Source: CAD feature listing. Evaluate the final solid. Frame: model axes, mm. Face numbers are marked on the shaded views. Give positions to 0.01 mm unless a question says otherwise; leave off trailing zeros. Order: outer loops, then holes, each group sorted by start corner. A loop starts at its lowest first (then second) coordinate and runs counter-clockwise, first axis right, second up.
from build123d import *

# Parameters (mm, degrees)
F0_R     = 1.2342692754
F0_R_2   = 1.7514332525
F0_R_3   = 1.6840139575
F0_R_4   = 0.6424379712
F0_R_5   = 0.6344814838
F1_DEPTH = 3.302


with BuildPart() as f1:
    # F0 (on Right) → F1 (new body)
    with BuildSketch(Plane.YZ):
        Polygon((30.1141384989, 0), (0, 0), (-32.9401008785, 0), (-32.9401008785, -0.8831103914), (-32.9401008785, -2.5610264856), (-32.9401008785, -3.4441391472), (-6.9765895605, -5.3869867697), (30.1141384989, -3.6207614467), (30.1141384989, -2.5610264856), (30.1141384989, -0.883640887), align=None)
        with Locations((-23.4924610704, -2.4733557366)):
            Circle(F0_R, mode=Mode.SUBTRACT)
        with Locations((-2.4024450686, -2.4733557366)):
            Circle(F0_R_2, mode=Mode.SUBTRACT)
        with Locations((3.7611864973, -2.4733557366)):
            Circle(F0_R_3, mode=Mode.SUBTRACT)
        Polygon((-32.9401008785, -2.5610264856), (-32.9401008785, -0.8831103914), (-35.3245027363, -0.8831103914), (-35.3245027363, -1.5608620106), (-35.3245027363, -1.7220684385), (-35.3245027363, -1.8952260725), (-35.3245027363, -2.5610264856), align=None)
        Polygon((32.4102304876, -0.883640887), (30.1141384989, -0.883640887), (30.1141384989, -2.5610264856), (32.4102304876, -2.5610264856), (32.4102304876, -1.8952260725), (32.4102304876, -1.7223336863), (32.4102304876, -1.5608620106), align=None)
        with BuildLine():
            Line((-35.3245027363, -1.7220684385), (-35.3245027363, -1.5608620106))
            Line((-35.3245027363, -1.5608620106), (-36.7480435846, -1.5608620106))
            ThreePointArc((-36.7480435846, -1.5608620106), (-36.7395622808, -1.6412672061), (-36.736718196, -1.7220684385))
            Line((-36.736718196, -1.7220684385), (-35.3245027363, -1.7220684385))
        make_face()
        with BuildLine():
            Line((34.18918825, -1.5608620106), (32.4102304876, -1.5608620106))
            Line((32.4102304876, -1.5608620106), (32.4102304876, -1.7223336863))
            Line((32.4102304876, -1.7223336863), (32.4102304876, -1.8952260725))
            Line((32.4102304876, -1.8952260725), (34.1978147229, -1.8702070236))
            ThreePointArc((34.1978147229, -1.8702070236), (34.1834682887, -1.7158143054), (34.18918825, -1.5608620106))
        make_face()
        with BuildLine():
            Line((-36.7497117243, -1.8952260725), (-35.3245027363, -1.8952260725))
            Line((-35.3245027363, -1.8952260725), (-35.3245027363, -1.7220684385))
            Line((-35.3245027363, -1.7220684385), (-36.736718196, -1.7220684385))
            ThreePointArc((-36.736718196, -1.7220684385), (-36.7367181732, -1.7222010624), (-36.7367181656, -1.7223336863))
            ThreePointArc((-36.7367181656, -1.7223336863), (-36.7399711292, -1.8090236652), (-36.7497117243, -1.8952260725))
        make_face()
        with BuildLine():
            ThreePointArc((-36.736718196, -1.7220684385), (-36.7395622808, -1.6412672061), (-36.7480435846, -1.5608620106))
            ThreePointArc((-36.7480435846, -1.5608620106), (-39.050204678, -1.7165627393), (-36.7497117243, -1.8952260725))
            ThreePointArc((-36.7497117243, -1.8952260725), (-36.7399711292, -1.8090236652), (-36.7367181656, -1.7223336863))
            ThreePointArc((-36.7367181656, -1.7223336863), (-36.7367181732, -1.7222010624), (-36.736718196, -1.7220684385))
        make_face()
        with Locations((-37.8934686196, -1.7223336863)):
            Circle(F0_R_4, mode=Mode.SUBTRACT)
        with BuildLine():
            Line((34.1978147229, -1.5608620106), (34.18918825, -1.5608620106))
            ThreePointArc((34.18918825, -1.5608620106), (34.1834682887, -1.7158143054), (34.1978147229, -1.8702070236))
            Line((34.1978147229, -1.8702070236), (34.1978147229, -1.5608620106))
        make_face()
        with BuildLine():
            ThreePointArc((36.5784095148, -1.6824278282), (35.4415677285, -0.4862718496), (34.18918825, -1.5608620106))
            Line((34.18918825, -1.5608620106), (34.1978147229, -1.5608620106))
            Line((34.1978147229, -1.5608620106), (34.1978147229, -1.8702070236))
            ThreePointArc((34.1978147229, -1.8702070236), (35.4748874223, -2.876422446), (36.5784095148, -1.6824278282))
        make_face()
        with Locations((35.3807061911, -1.6824278282)):
            Circle(F0_R_5, mode=Mode.SUBTRACT)
    extrude(amount=F1_DEPTH)


solid = f1.part
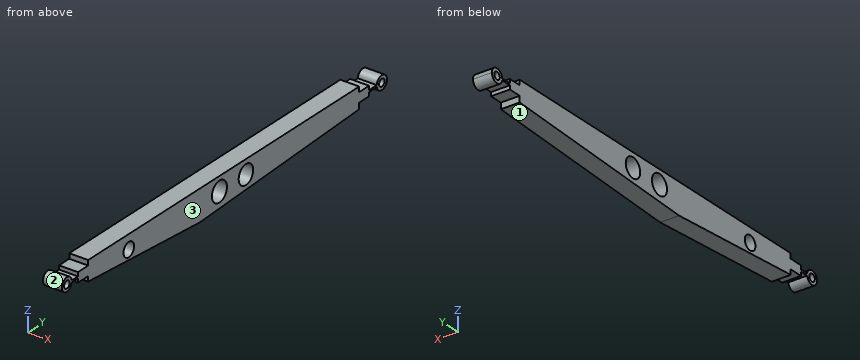
1) Section query C-C on y = -20.5. Output: boundary loops of the cut face in (x, z).
Checks:
outline: (0, -4.38) - (3.3, -4.38) - (3.3, 0) - (0, 0) - close
2) Pull-direction query (Y, two-part tool) for the marked faces 1, 2 and 3; classes: +Y half, -Y half, draft (parallel to the pull), parting line (faces both ways), or undercut.
Checks:
face 1: +Y half
face 2: undercut
face 3: draft
3) Ray query, L1, parallel to Y at x = 3, z = -1; L2, parallel to Y at x = 1.7, z = -1.65; L3, parallel to Z at x = 0.7, y = -33. Return the intervals inside material, ascending.
Checks:
L1: y = -38.8 to -36.99, -35.32 to -3.35, -1.46 to 2.95, 4.58 to 32.41, 34.4 to 36.36
L2: y = -39.05 to -38.53, -37.26 to -24.41, -22.57 to -3.95, -0.86 to 2.29, 5.23 to 34.75, 36.01 to 36.58
L3: z = -2.56 to -0.88
4) Section query B-B on y = -32. Output: boundary loops of the cut face in (x, z), and give its area (3 significant figures).
Checks:
outline: (0, -3.51) - (3.3, -3.51) - (3.3, 0) - (0, 0) - close
area: 11.6 mm2
5) First-contact query: pin 1 Ø1.9 at (x, y) = (1, -34) entering from -Z; pin 2 Ø1 at (x, z) = (1.5, -0.5) entering from -Y; pin 3 Ø0.7 at (x, z) = (1, -2.5) entering from -Y. Flat tips, straight axial feed; report the tip coordinate or a pass-through.
Checks:
pin 1: stops at z = -2.56
pin 2: stops at y = -38.8
pin 3: stops at y = -38.97
6) Section query A-A on x = 2. Output: boundary loops of the cut face in (y, z).
Checks:
outline: (-36.75, -1.9) - (-35.32, -1.9) - (-35.32, -2.56) - (-32.94, -2.56) - (-32.94, -3.44) - (-6.98, -5.39) - (30.11, -3.62) - (30.11, -2.56) - (32.41, -2.56) - (32.41, -1.9) - (34.2, -1.87) arc R1.2 ccw (long way) to (34.19, -1.56) - (32.41, -1.56) - (32.41, -0.88) - (30.11, -0.88) - (30.11, 0) - (-32.94, 0) - (-32.94, -0.88) - (-35.32, -0.88) - (-35.32, -1.56) - (-36.75, -1.56) arc R1.16 ccw (long way) to start; hole circle Ø1.28 at (-37.89, -1.72); hole circle Ø2.47 at (-23.49, -2.47); hole circle Ø3.5 at (-2.4, -2.47); hole circle Ø3.37 at (3.76, -2.47); hole circle Ø1.27 at (35.38, -1.68)
